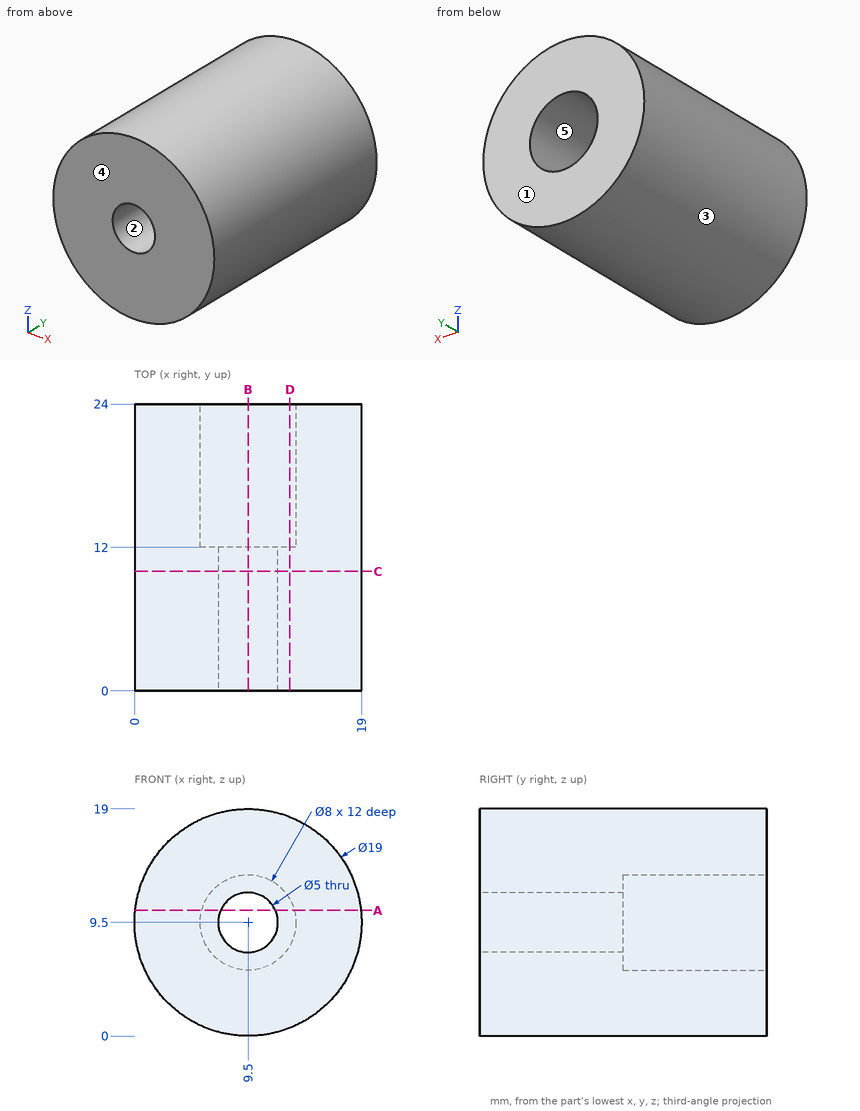
Drawing for the job (mm, zero at the part's lowest x, y, z). A direction names the side the tool comes from. Coordinates: 2 decimals unless noted, no trailing zeros. Order: outer loops, then holes, each group sorted by start corner. A loop starts at its lowest first (then second) coordinate and runs counter-clockwise, first axis right, second up. Notation, with made-up numbers: (-25.5, 6.25) - (-15.5, 6.25) arc R19 cw to (-15.5, 10.25) - close; hole circle Ø2 at (-7.75, 86.5). An arc over 180 degrees is marked (long way). Use a Markdown table: item, result. Add a question column.
(1) Saw through at D-D (x = 13). Give the cut face in (y, z), then the cut area to 3 significant figures.
(2) Flat gauge pins, fed straight in: pin 1 (5 mm diameter, centred on y = 18.5, z = 16, fed in from -X); pin 2 (4 mm diameter, centred on y = 18, z = 3.5, fed in from +X); pin 3 (1 mm diameter, centred on x = 17, y = 6, fed in from +Z). Where does each tip first touch, or does it go through?
(3) Pull direction X, two halves, no side cores. Call the marked faces 1, 2 and 3: +X half, -X half, draft (parallel to the pull), parting line (faces both ways), or undercut.
(4) Saw through at C-C (y = 10). Give the cut face in (x, z), then the cut area to 3 significant figures.
(5) Saw through at A-A (z = 10.5). Give the cut face in (x, y).
(6) Which spindle directions (+Z, -Z, +X, -X, +Y, -Y) get a long thin tool onto all of the face, cutting with end or side? Do the marked faces 4 and 5. Say none if no direction does.
(7) Drill centre lines: line 1 along X through (y, z) = (14.75, 9.5); line 2 along Z through (x, y) = (9.5, 5.25). Where is each one in solid material? Low to high. Write a range as [from, to].
(8) Saw through at B-B (x = 9.5). Give the cut face in (y, z).
Solved:
| question | item | result |
|---|---|---|
| 1 | outline | (0, 0.67) - (24, 0.67) - (24, 7.56) - (12, 7.56) - (12, 11.44) - (24, 11.44) - (24, 18.33) - (0, 18.33) - close |
| 1 | area | 377 mm² |
| 2 | pin 1 | stops at x = 0.88 |
| 2 | pin 2 | stops at x = 18.12 |
| 2 | pin 3 | stops at z = 15.92 |
| 3 | face 1 | draft |
| 3 | face 2 | undercut |
| 3 | face 3 | parting line |
| 4 | outline | circle Ø19 at (9.5, 9.5); hole circle Ø5 at (9.5, 9.5) |
| 4 | area | 264 mm² |
| 5 | outline | (0.05, 0) - (7.21, 0) - (7.21, 12) - (5.63, 12) - (5.63, 24) - (0.05, 24) - close; (11.79, 0) - (18.95, 0) - (18.95, 24) - (13.37, 24) - (13.37, 12) - (11.79, 12) - close |
| 6 | face 4 | +Z, -Z, +X, -X, -Y |
| 6 | face 5 | +Y |
| 7 | line 1 | x = [0, 5.5], [13.5, 19] |
| 7 | line 2 | z = [0, 7], [12, 19] |
| 8 | outline | (0, 0) - (24, 0) - (24, 5.5) - (12, 5.5) - (12, 7) - (0, 7) - close; (0, 12) - (12, 12) - (12, 13.5) - (24, 13.5) - (24, 19) - (0, 19) - close |
